```python
from build123d import *

# Parameters (mm, degrees)
F1_DEPTH = 6


with BuildPart() as f1:
    # F0 (on Top) → F1 (new body)
    with BuildSketch(Plane.XY):
        Polygon((1000, 0), (0, 0), (0, -63.39746), (26.905989, -110), (73.094011, -110), (100, -63.39746), (126.905989, -110), (173.094011, -110), (200, -63.39746), (226.905989, -110), (273.094011, -110), (300, -63.39746), (326.905989, -110), (373.094011, -110), (400, -63.39746), (426.905989, -110), (473.094011, -110), (500, -63.39746), (526.905989, -110), (573.094011, -110), (600, -63.39746), (626.905989, -110), (673.094011, -110), (700, -63.39746), (726.905989, -110), (773.094011, -110), (800, -63.39746), (826.905989, -110), (873.094011, -110), (900, -63.39746), (926.905989, -110), (973.094011, -110), (1000, -63.39746), align=None)
        Polygon((26.905989, -110), (0, -63.39746), (0, -110), align=None)
        Polygon((1000, -110), (1000, -63.39746), (973.094011, -110), align=None)
        Polygon((73.094011, -110), (26.905989, -110), (50, -150), align=None)
        Polygon((950, -150), (973.094011, -110), (926.905989, -110), align=None)
        Polygon((100, -63.39746), (73.094011, -110), (126.905989, -110), align=None)
        Polygon((873.094011, -110), (926.905989, -110), (900, -63.39746), align=None)
        Polygon((173.094011, -110), (126.905989, -110), (150, -150), align=None)
        Polygon((850, -150), (873.094011, -110), (826.905989, -110), align=None)
        Polygon((200, -63.39746), (173.094011, -110), (226.905989, -110), align=None)
        Polygon((773.094011, -110), (826.905989, -110), (800, -63.39746), align=None)
        Polygon((273.094011, -110), (226.905989, -110), (250, -150), align=None)
        Polygon((750, -150), (773.094011, -110), (726.905989, -110), align=None)
        Polygon((300, -63.39746), (273.094011, -110), (326.905989, -110), align=None)
        Polygon((673.094011, -110), (726.905989, -110), (700, -63.39746), align=None)
        Polygon((373.094011, -110), (326.905989, -110), (350, -150), align=None)
        Polygon((650, -150), (673.094011, -110), (626.905989, -110), align=None)
        Polygon((400, -63.39746), (373.094011, -110), (426.905989, -110), align=None)
        Polygon((573.094011, -110), (626.905989, -110), (600, -63.39746), align=None)
        Polygon((473.094011, -110), (426.905989, -110), (450, -150), align=None)
        Polygon((550, -150), (573.094011, -110), (526.905989, -110), align=None)
        Polygon((500, -63.39746), (473.094011, -110), (526.905989, -110), align=None)
    extrude(amount=F1_DEPTH)


solid = f1.part
```
The listing builds one solid part. Answer for the finished solid, in the listing's coordinates (mm). A direction names the side the tool comes from. Give positions to 0.01 mm unless a question says otherwise; leave off trailing zeros. Write each loop counter-clockwise with the first axis right and the second up, starting at its lowest first coordinate (ties: lowest second). Pieces come first, ordered by that corner, then holes. Notation, with made-up numbers: M 38,69.5 L 75,69.5 A37 cw 75,106.5 Z; hole C 6,-2.75 d4. An arc over 180 degrees is marked long. Write each question's results on one line, items separated by ' | '.
Q1. Section C-C, the plane y = -137 is taken. Count the separate pieces of the cut face and the enclosed holes in it, then the cut area to 3 significant figures.
Output values:
separate pieces: 10 | enclosed holes: 0 | area: 901 mm2
Q2. Consider L1, parallel to Y at x = 386, z = 2.9; L2, parallel to Y at x = 327, z = 5.4. Determine where each line is inside the solid, lowest interval first. Write a range as from..to.
Output values:
L1: -110..0 | L2: -110.16..0
Q3. Section D-D, the plane x = 537.5 is taken. Write down the section's boundary in (y, z).
Output values:
outline: M -128.35,0 L 0,0 L 0,6 L -128.35,6 Z
Q4. For a pull along X with two mould halves and no side action, classify faces 3 (the flat face through (38.29, -129.72, 2.96)), 4 (the flat face through (61.385, -130.28, 2.958)), 5 (the flat face through (493, -57, 0)) as released by +X, released by -X, zero draft, split by the parting line, or undercut.
Output values:
face 3: released by -X | face 4: undercut | face 5: zero draft
Q5. A flat-ended cylindrical pin translates along its axis: P1, Ø1.8, axis at x = 813, z = 1.5, coming from the -Y side. Find the tip coordinate at first contact, or state that the pin passes through.
Output values:
P1: y = -110
Q6. Section B-B, the plane x = 208 is taken. Write down the section's boundary in (y, z), then the cut area to 3 significant figures.
Output values:
outline: M -110,0 L 0,0 L 0,6 L -110,6 Z | area: 660 mm2
Q7. A tool of negligible diameter and unlimited length cuts with its end or side. For faces 1 (the flat face through (138.29, -129.72, 2.96)), 2 (the flat face through (961.385, -130.28, 2.958)), from which of +Z, -Z, +X, -X, +Y, -Y can it reach the whole face along a straight path? Write none if from no direction.
Output values:
face 1: +Z, -Z, -Y | face 2: +Z, -Z, +X, -Y
